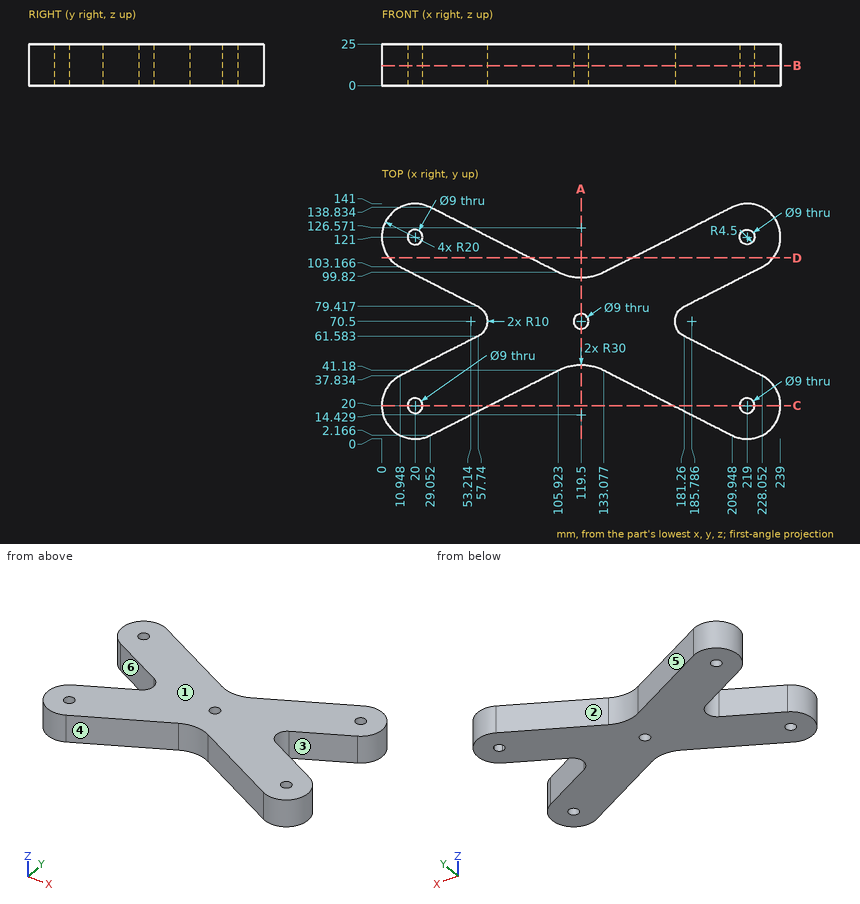
Source: three-view drawing plus pictorial views. Frame: mm from the lowest corner of the part. A direction names the side the tool comes from. Round coordinates to 2 decimals unless told otherwise and drop trailing zeros. Loops run counter-clockwise (first coordinate to the right, second up) from the corner with the lowest first, then second, coordinate; pieces in that order, holes last.
Q1. Access query for the marked faces 4, 5 and 6. Directions: +Z, -Z, +X, -X, +Y, -Y. A direction counts if a zero-diameter tool reaches every point of the face in a straight line with its end or side. Return the directions, or none.
Q2. First-contact query: P1, Ø11.5, axis at x = 219, y = 121, coming from the -Z side; P2, Ø6, axis at x = 52, z = 13, coming from the +Y side; P3, Ø4, axis at x = 109, z = 18, coming from the -Y side; P4, Ø10, axis at x = 165, z = 17, coming from the +Y side. Flat tips, straight axial feed; report the tip coordinate or a pass-through.
Q3. Section B-B, the plane z = 12. Return loops of the section in (x, y) (1 decimal).
Q4. Section C-C, the plane y = 20. Return loops of the section in (x, z).
Q5. Mould query, pull axis X, two halves, no side actions, for the marked faces 1, 2 and 3. Classes: pulls with the +X half, pulls with the -X half, needs draft (parallel to the pull), parting line crosses it, or undercut.
Q6. Ray query, line 1 (X direction, y = 121, z = 7.75) (1 decimal); line 2 (Y direction, x = 20, z = 17); line 3 (Y direction, x = 218.5, z = 17.75) (1 decimal). Return the intervals inside material, ascending.
Q7. Section A-A, the plane x = 119.5. Return loops of the section in (y, z), plus the area to 3 significant figures.
Q8. Section D-D, the plane y = 108.5. Return loops of the section in (x, z), plus the area to 3 significant figures.
Solutions:
1. face 4: +Z, -Z, -Y
1. face 5: +Z, -Z, +Y
1. face 6: +Z, -Z, -X
2. P1: stops at z = 0
2. P2: stops at y = 128.71
2. P3: stops at y = 41.7
2. P4: stops at y = 118.56
3. outline: (10.9, 37.8) arc R20 ccw to (29.1, 2.2) - (105.9, 41.2) arc R30 cw to (133.1, 41.2) - (209.9, 2.2) arc R20 ccw to (228.1, 37.8) - (181.3, 61.6) arc R10 cw to (181.3, 79.4) - (228.1, 103.2) arc R20 ccw to (209.9, 138.8) - (133.1, 99.8) arc R30 cw to (105.9, 99.8) - (29.1, 138.8) arc R20 ccw to (10.9, 103.2) - (57.7, 79.4) arc R10 cw to (57.7, 61.6) - close; hole circle Ø9 at (20, 20); hole circle Ø9 at (20, 121); hole circle Ø9 at (119.5, 70.5); hole circle Ø9 at (219, 20); hole (219, 116.5) arc R4.5 ccw to (223.5, 121) arc R4.5 ccw (long way) to start
4. outline: (0, 0) - (15.5, 0) - (15.5, 25) - (0, 25) - close; (24.5, 0) - (64.19, 0) - (64.19, 25) - (24.5, 25) - close; (174.81, 0) - (214.5, 0) - (214.5, 25) - (174.81, 25) - close; (223.5, 0) - (239, 0) - (239, 25) - (223.5, 25) - close
5. face 1: needs draft
5. face 2: undercut
5. face 3: pulls with the +X half
6. line 1: x = 0 to 15.5, 24.5 to 64.2, 174.8 to 214.5, 223.5 to 239
6. line 2: y = 0 to 15.5, 24.5 to 42.43, 98.57 to 116.5, 125.5 to 141
6. line 3: y = 0 to 15.5, 24.5 to 42.7, 98.3 to 116.5, 125.5 to 141
7. outline: (44.43, 0) - (66, 0) - (66, 25) - (44.43, 25) - close; (75, 0) - (96.57, 0) - (96.57, 25) - (75, 25) - close
7. area: 1,080 mm2
8. outline: (4.39, 0) - (88.82, 0) - (88.82, 25) - (4.39, 25) - close; (150.18, 0) - (234.61, 0) - (234.61, 25) - (150.18, 25) - close
8. area: 4,220 mm2
